```python
from build123d import *

# Parameters (mm, degrees)
SKETCH_W            = 440
SKETCH_H            = 50
PAD_DEPTH           = 5
SKETCH001_R         = 17.5
POCKET_DEPTH        = 1
FILLET_R            = 5
LINEARPATTERN_COUNT = 6
LINEARPATTERN_PITCH = 65


with BuildPart() as part:
    # Sketch → Pad (new body)
    with BuildSketch(Plane.XY):
        with Locations((147.117165, 35.792885)):
            Rectangle(SKETCH_W, SKETCH_H)
    extrude(amount=PAD_DEPTH)

    # Sketch001 (on Face6 of Pad) → Pocket (cut)
    with BuildSketch(Plane.XY.offset(5)):
        with Locations((-15.382835, 35.792885)):
            Circle(SKETCH001_R)
    pocket = extrude(amount=-POCKET_DEPTH, mode=Mode.SUBTRACT)

    # Fillet
    fillet_edges = [part.edges().sort_by_distance(p)[0] for p in [
        (-72.882835, 10.792885, 2.5),
        (367.117165, 10.792885, 2.5),
        (367.117165, 60.792885, 2.5),
        (-72.882835, 60.792885, 2.5),
    ]]
    fillet(fillet_edges, radius=FILLET_R)

    # LinearPattern: Pocket ×6
    with Locations(*[(i * LINEARPATTERN_PITCH, 0, 0) for i in range(1, LINEARPATTERN_COUNT)]):
        add(pocket, mode=Mode.SUBTRACT)


solid = part.part
```
Geometry check sheet. Reference: the model listing, model coordinates, mm. A direction names the side the tool comes from. Round coordinates to 2 decimals unless told otherwise and drop trailing zeros. Order: outer loops, then holes, each group sorted by start corner. A loop starts at its lowest first (then second) coordinate and runs counter-clockwise, first axis right, second up. Notation, with made-up numbers: (-30.5, 25.5) -> (-19.5, 25.5) arc R32 cw to (-19.5, 60.5) -> close; hole circle Ø1 at (49, 45). An arc over 180 degrees is marked (long way). Return JSON: item names as keys, results as strings. Group by question number.
Q1. Section check C-C, the plane x = 241. Record the boundary of the cut face in (y, z), plus the area to 3 significant figures.
Q2. Section check A-A, the plane x = 319. Record the boundary of the cut face in (y, z), plus the area to 3 significant figures.
Q3. Gauge pin test, flat ends, axial feed: pin 1 (21 mm diameter, centred on x = -15.38, y = 35.79, fed in from +Z); pin 2 (5 mm diameter, centred on x = 142.5, y = 24, fed in from -Z). Record the tip position at first contact, or that the pin passes through.
Q4. Release check for a two-part mould opening along Y. For faces 1 (the flat face through (144, 36, 0)), 2 (the cylindrical face through (130.783, 29.09, 4.507)) record: released by +Y, released by -Y, zero draft, split by the parting line, or undercut.
Q5. Tool access check on faces 3 (the flat face through (244, 36, 4)), 4 (the flat face through (144, 36, 5)). Record the directions out of +Z, -Z, +X, -X, +Y, -Y that give a thin tool (end or side, any length) a straight path to the whole face; none if there is none.
Q6. Material ranges on probe 1 along Z at (x, y) = (169, 48); probe 2 along Y at (x, z) = (185.5, 4.05); probe 3 along X at (y, z) = (58.5, 0.3), recorded low to high. Write a range as from..to.
Q7. Section check B-B, the plane y = 32. Record the boundary of the cut face in (x, z), plus the area to 3 significant figures.
Q8. Section check D-D, the plane y = 48. Record the boundary of the cut face in (x, z), plus the area to 3 significant figures.
Numbers:
{
 "1": {"outline": "(10.79, 0) -> (60.79, 0) -> (60.79, 5) -> (52.91, 5) -> (52.91, 4) -> (18.67, 4) -> (18.67, 5) -> (10.79, 5) -> close", "area": "216 mm^2"},
 "2": {"outline": "(10.79, 0) -> (60.79, 0) -> (60.79, 5) -> (50.56, 5) -> (50.56, 4) -> (21.02, 4) -> (21.02, 5) -> (10.79, 5) -> close", "area": "220 mm^2"},
 "3": {"pin 1": "z = 4", "pin 2": "z = 0"},
 "4": {"face 1": "zero draft", "face 2": "undercut"},
 "5": {"face 3": "+Z", "face 4": "+Z, +X, -X, +Y, -Y"},
 "6": {"probe 1": "0..4", "probe 2": "10.79..19.31, 52.27..60.79", "probe 3": "-72.09..366.32"},
 "7": {"outline": "(-72.88, 0) -> (367.12, 0) -> (367.12, 5) -> (326.7, 5) -> (326.7, 4) -> (292.53, 4) -> (292.53, 5) -> (261.7, 5) -> (261.7, 4) -> (227.53, 4) -> (227.53, 5) -> (196.7, 5) -> (196.7, 4) -> (162.53, 4) -> (162.53, 5) -> (131.7, 5) -> (131.7, 4) -> (97.53, 4) -> (97.53, 5) -> (66.7, 5) -> (66.7, 4) -> (32.53, 4) -> (32.53, 5) -> (1.7, 5) -> (1.7, 4) -> (-32.47, 4) -> (-32.47, 5) -> (-72.88, 5) -> close", "area": "1,990 mm^2"},
 "8": {"outline": "(-72.88, 0) -> (367.12, 0) -> (367.12, 5) -> (322.16, 5) -> (322.16, 4) -> (297.08, 4) -> (297.08, 5) -> (257.16, 5) -> (257.16, 4) -> (232.08, 4) -> (232.08, 5) -> (192.16, 5) -> (192.16, 4) -> (167.08, 4) -> (167.08, 5) -> (127.16, 5) -> (127.16, 4) -> (102.08, 4) -> (102.08, 5) -> (62.16, 5) -> (62.16, 4) -> (37.08, 4) -> (37.08, 5) -> (-2.84, 5) -> (-2.84, 4) -> (-27.92, 4) -> (-27.92, 5) -> (-72.88, 5) -> close", "area": "2,050 mm^2"}
}
